Check sheet for the drawn part. Datum: minimum x, y, z corner. Units: mm. A direction names the side the tool comes from. Give positions to 0.01 mm unless a question says otherwise; leave off trailing zeros. Loops run counter-clockwise (first coordinate to the right, second up) from the corner with the lowest first, then second, coordinate; pieces in that order, holes last.
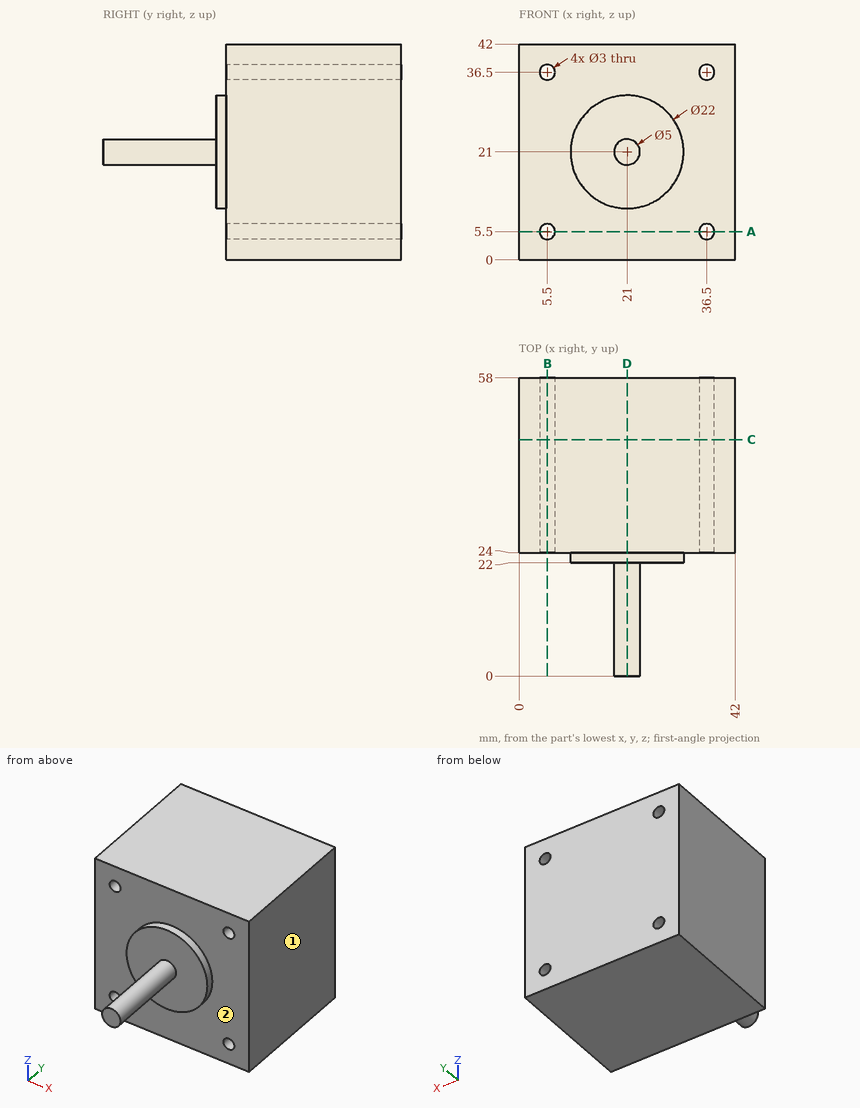
(1) Section check D-D on x = 21. Record the boundary of the cut face in (y, z).
(2) Access from +Z, -Z, +X, -X, +Y, -Y to the whole of each face (thin tool, end or side, straight path). Record for the marked faces 1 and 2.
(3) Section check A-A on z = 5.5. Record the boundary of the cut face in (x, y).
(4) Section check C-C on y = 46. Record the boundary of the cut face in (x, z), plus the area to 3 significant figures.
(5) Material ranges on line 1 (Z direction, x = 5.5, y = 49.5); line 2 (X direction, y = 34, z = 35.5); line 3 (Z direction, x = 36, y = 39), recorded low to high.
(6) Gauge pin test, flat ends, axial feed: pin 1 Ø5 at (x, y) = (27, 13.5) entering from -Z; pin 2 Ø1 at (x, z) = (9, 17.5) entering from -Y; pin 3 Ø4 at (y, z) = (12.5, 22.5) entering from +X; pin 4 Ø10 at (x, z) = (22.5, 11) entering from -Y. Record the tip position at first contact, or that the pin passes through.
(7) Section check B-B on x = 5.5. Record the boundary of the cut face in (y, z), plus the area to 3 significant figures.
Computed values:
1. outline: (0, 18.5) - (22, 18.5) - (22, 10) - (24, 10) - (24, 0) - (58, 0) - (58, 42) - (24, 42) - (24, 32) - (22, 32) - (22, 23.5) - (0, 23.5) - close
2. face 1: +Z, -Z, +X, +Y, -Y
2. face 2: -Y
3. outline: (0, 24) - (4, 24) - (4, 58) - (0, 58) - close; (7, 24) - (35, 24) - (35, 58) - (7, 58) - close; (38, 24) - (42, 24) - (42, 58) - (38, 58) - close
4. outline: (0, 0) - (42, 0) - (42, 42) - (0, 42) - close; hole circle Ø3 at (5.5, 5.5); hole circle Ø3 at (5.5, 36.5); hole circle Ø3 at (36.5, 5.5); hole circle Ø3 at (36.5, 36.5)
4. area: 1,740 mm2
5. line 1: z = 0 to 4, 7 to 35, 38 to 42
5. line 2: x = 0 to 4.38, 6.62 to 35.38, 37.62 to 42
5. line 3: z = 0 to 4.09, 6.91 to 35.09, 37.91 to 42
6. pin 1: passes through
6. pin 2: stops at y = 24
6. pin 3: stops at x = 23.5
6. pin 4: stops at y = 22
7. outline: (24, 0) - (58, 0) - (58, 4) - (24, 4) - close; (24, 7) - (58, 7) - (58, 35) - (24, 35) - close; (24, 38) - (58, 38) - (58, 42) - (24, 42) - close
7. area: 1,220 mm2
